```python
from build123d import *

# Parameters (mm, degrees)
SKETCH1_W           = 12
SKETCH1_H           = 248
BOSS_EXTRUDE1_DEPTH = 0.5
SKETCH2_W           = 5
SKETCH2_H           = 5
BOSS_EXTRUDE2_DEPTH = 1


with BuildPart() as part:
    # Sketch1 → Boss-Extrude1 (new body)
    with BuildSketch(Plane.XY):
        Rectangle(SKETCH1_W, SKETCH1_H)
    extrude(amount=BOSS_EXTRUDE1_DEPTH)

    # Sketch2 → Boss-Extrude2 (add)
    with BuildSketch(Plane.XY.offset(0.5)):
        with Locations((0, -120.5)):
            Rectangle(SKETCH2_W, SKETCH2_H)
        with Locations((0, -113.67)):
            Rectangle(SKETCH2_W, SKETCH2_H)
        with Locations((0, -106.84)):
            Rectangle(SKETCH2_W, SKETCH2_H)
        with Locations((0, -100.01)):
            Rectangle(SKETCH2_W, SKETCH2_H)
        with Locations((0, -93.18)):
            Rectangle(SKETCH2_W, SKETCH2_H)
        with Locations((0, -86.35)):
            Rectangle(SKETCH2_W, SKETCH2_H)
        with Locations((0, -79.52)):
            Rectangle(SKETCH2_W, SKETCH2_H)
        with Locations((0, -72.69)):
            Rectangle(SKETCH2_W, SKETCH2_H)
        with Locations((0, -65.86)):
            Rectangle(SKETCH2_W, SKETCH2_H)
        with Locations((0, -59.03)):
            Rectangle(SKETCH2_W, SKETCH2_H)
        with Locations((0, -52.2)):
            Rectangle(SKETCH2_W, SKETCH2_H)
        with Locations((0, -45.37)):
            Rectangle(SKETCH2_W, SKETCH2_H)
        with Locations((0, -38.54)):
            Rectangle(SKETCH2_W, SKETCH2_H)
        with Locations((0, -31.71)):
            Rectangle(SKETCH2_W, SKETCH2_H)
        with Locations((0, -24.88)):
            Rectangle(SKETCH2_W, SKETCH2_H)
        with Locations((0, -18.05)):
            Rectangle(SKETCH2_W, SKETCH2_H)
        with Locations((0, -11.22)):
            Rectangle(SKETCH2_W, SKETCH2_H)
        with Locations((0, -4.39)):
            Rectangle(SKETCH2_W, SKETCH2_H)
        with Locations((0, 2.44)):
            Rectangle(SKETCH2_W, SKETCH2_H)
        with Locations((0, 9.27)):
            Rectangle(SKETCH2_W, SKETCH2_H)
        with Locations((0, 16.1)):
            Rectangle(SKETCH2_W, SKETCH2_H)
        with Locations((0, 22.93)):
            Rectangle(SKETCH2_W, SKETCH2_H)
        with Locations((0, 29.76)):
            Rectangle(SKETCH2_W, SKETCH2_H)
        with Locations((0, 36.59)):
            Rectangle(SKETCH2_W, SKETCH2_H)
        with Locations((0, 43.42)):
            Rectangle(SKETCH2_W, SKETCH2_H)
        with Locations((0, 50.25)):
            Rectangle(SKETCH2_W, SKETCH2_H)
        with Locations((0, 57.08)):
            Rectangle(SKETCH2_W, SKETCH2_H)
        with Locations((0, 63.91)):
            Rectangle(SKETCH2_W, SKETCH2_H)
        with Locations((0, 70.74)):
            Rectangle(SKETCH2_W, SKETCH2_H)
        with Locations((0, 77.57)):
            Rectangle(SKETCH2_W, SKETCH2_H)
        with Locations((0, 84.4)):
            Rectangle(SKETCH2_W, SKETCH2_H)
        with Locations((0, 91.23)):
            Rectangle(SKETCH2_W, SKETCH2_H)
        with Locations((0, 98.06)):
            Rectangle(SKETCH2_W, SKETCH2_H)
        with Locations((0, 104.89)):
            Rectangle(SKETCH2_W, SKETCH2_H)
        with Locations((0, 111.72)):
            Rectangle(SKETCH2_W, SKETCH2_H)
        with Locations((0, 118.55)):
            Rectangle(SKETCH2_W, SKETCH2_H)
    extrude(amount=BOSS_EXTRUDE2_DEPTH)


solid = part.part
```
The listing builds one solid part. Answer for the finished solid, in the listing's coordinates (mm). Give positions to 0.01 mm unless a question says otherwise; leave off trailing zeros. Answer as CSV lines item,"result". Start each with the question number.
Q1. Given pin 1 (0.5 mm diameter, centred on x = 0, z = 1, fed in from +Y); pin 2 (1.5 mm diameter, centred on x = -3.5, y = 72, fed in from +Z); pin 3 (0.8 mm diameter, centred on x = 0.5, z = 1, fed in from -Y), each flat-ended and moving along its own axis, determine where each tip first touches the part or whether it passes through.
Q2. A cutting plane is placed at A-A (z = 1.1). Count the separate pieces of the cut face and the enclosed holes in it, then the cut area to 3 significant figures.
Q3. Find the intervals of material crossed by L1, parallel to X at y = 70, z = 0.95; L2, parallel to Z at x = 4, y = 68.5, in increasing order.
Results found:
1,pin 1,"y = 121.05"
1,pin 2,"z = 0.5"
1,pin 3,"y = -123"
2,separate pieces,"36"
2,enclosed holes,"0"
2,area,"900 mm2"
3,L1,"-2.5 to 2.5"
3,L2,"0 to 0.5"
